Verification items for the finished model (mm, model axes). Face numbers are marked on the shaded views. A direction names the side the tool comes from. Round coordinates to 2 decimals unless told otherwise and drop trailing zeros. Write each loop counter-clockwise with the first axis right and the second up, starting at its lowest first coordinate (ties: lowest second). Pieces come first, ordered by that corner, then holes. Notation, with made-up numbers: (40, 73.5) -> (56, 73.5) arc R27 cw to (56, 111.5) -> close; hole circle Ø7 at (58, -4). An arc over 180 degrees is marked (long way). Answer as a JSON object with one key per item and string values. Group by question number.
(1) Set-up check for the marked faces 1, 2, 3, 4 and 5: record each of +Z, -Z, +X, -X, +Y, -Y from which the full face is reachable in a straight line by a thin tool's end or side.
(2) Sectioned sample at C-C on z = -1.5. Record the cut outline in (x, y).
(3) Gauge pin test, flat ends, axial feed: pin 1 Ø4.5 at (x, y) = (7.5, -19.5) entering from +Z; pin 2 Ø5 at (x, z) = (3, -15) entering from -Y; pin 3 Ø3 at (x, z) = (15.5, -7) entering from -Y; pin 4 Ø10 at (x, y) = (16.5, 34) entering from -Z. Record the tip position at first contact, or that the pin passes through.
(4) Scan lines: L1, parallel to X at y = 11, z = -17; L2, parallel to Y at x = 13, z = 2; L3, parallel to Z at x = 5.25, y = 18. Record each from-to range of solid material in increasing order. Write a range as from..to.
(5) Draft check along Z on the marked faces 6 and 7. Enter one of: released by +Z, released by -Z, zero draft, split by the parting line, or undercut.
(6) Sectioned sample at B-B on y = 49.5. Record the cut outline in (x, z), and give its area (3 significant figures).
(7) Sectioned sample at D-D on x = 16. Record the cut outline in (y, z), and give its area (3 significant figures).
```python
from build123d import *

# Parameters (mm, degrees)
BOSS_EXTRUDE1_DEPTH     = 50
CUT_EXTRUDE1_DEPTH      = 30
BOSS_EXTRUDE2_DEPTH     = 2
CUT_EXTRUDE2_DEPTH      = 2
CUT_EXTRUDE3_DEPTH      = 2
SKETCH9_W               = 3
SKETCH9_H               = 16.82
BOSS_EXTRUDE3_DEPTH     = 13
SKETCH10_W              = 4
SKETCH10_H              = 4
CUT_EXTRUDE4_DEPTH      = 15
BOSS_EXTRUDE4_DEPTH     = 8.82
FILLET1_R               = 1.5
SKETCH12_R              = 0.75
CUT_EXTRUDE5_DEPTH      = 57.090755147
CUT_EXTRUDE7_DEPTH      = 58.56944687
CUT_EXTRUDE7_DEPTH_BACK = 58.56944687
SKETCH15_R              = 0.75
BOSS_EXTRUDE5_DEPTH     = 7.6
CUT_EXTRUDE8_DEPTH      = 3
CUT_EXTRUDE9_DEPTH      = 3
SCALE1_SCALE            = 1.3


with BuildPart() as part:
    # Sketch1 → Boss-Extrude1 (new body)
    with BuildSketch(Plane(origin=(0, 0, 0), x_dir=(1, 0, 0), z_dir=(0, 1, 0))):
        Polygon((0, 0), (0, 16.82), (7.855052448, 23.008549995), (9.003996979, 21.550208451), (3, 16.82), (3, 0), (8.997095559, -4.738955219), (7.846023294, -6.199993425), align=None)
    extrude(amount=BOSS_EXTRUDE1_DEPTH)

    # Sketch2 → Cut-Extrude1 (cut, along a direction that is not the sketch's normal)
    with BuildSketch(Plane(origin=(0, 0, 0), x_dir=(0.7846023293722103, 0, 0.6199993425348946), z_dir=(-0.6199993425348946, 0, 0.7846023293722103))):
        Polygon((11.46, 50), (0, 37), (0, 50), align=None)
    extrude(amount=-CUT_EXTRUDE1_DEPTH, dir=(0, 0, 1), mode=Mode.SUBTRACT)

    # Sketch5 → Boss-Extrude2 (add, along a direction that is not the sketch's normal)
    with BuildSketch(Plane(origin=(-17.310263861, 11.972767428, 0), x_dir=(0, 0, 1), z_dir=(-0.8224425153975565, 0.568848230081223, 0))):
        Polygon((0, 30.43037307), (6.199993425, 44.223196672), (4.746003384, 46.236948917), (-21.566016526, 46.236948917), (-23.008549995, 44.239069366), (-16.82, 30.43037307), align=None)
    extrude(amount=BOSS_EXTRUDE2_DEPTH, dir=(0, 1, 0))

    # Sketch6 → Cut-Extrude2 (cut)
    with BuildSketch(Plane(origin=(0, 0, 0), x_dir=(0.7846023293722103, 0, 0.6199993425348946), z_dir=(-0.6199993425348946, 0, 0.7846023293722103))):
        Polygon((10, 50.343804538), (7, 0), (10, 0), align=None)
    extrude(amount=-CUT_EXTRUDE2_DEPTH, mode=Mode.SUBTRACT)

    # Sketch7 → Cut-Extrude3 (cut)
    with BuildSketch(Plane(origin=(-8.176434921, 0, -10.378250996), x_dir=(-0.7855052448151816, 0, 0.6188549994690533), z_dir=(-0.6188549994690533, 0, -0.7855052448151816))):
        Polygon((-20.409141091, 50.356858917), (-20.409141091, 0), (-17.409141091, 0), align=None)
    extrude(amount=-CUT_EXTRUDE3_DEPTH, mode=Mode.SUBTRACT)

    # Sketch9 → Boss-Extrude3 (add, along a direction that is not the sketch's normal)
    with BuildSketch(Plane.XZ):
        with Locations((1.5, -8.41)):
            Rectangle(SKETCH9_W, SKETCH9_H)
    extrude(amount=BOSS_EXTRUDE3_DEPTH, dir=(0.5000000000000012, -0.866025403784438, 0))

    # Sketch10 → Cut-Extrude4 (cut, along a direction that is not the sketch's normal)
    with BuildSketch(Plane(origin=(0, 0, 0), x_dir=(0, 0, 1), z_dir=(-0.8660254037844379, -0.5000000000000014, 0))):
        with Locations((-14.82, -11)):
            Rectangle(SKETCH10_W, SKETCH10_H)
        with Locations((-2, -11)):
            Rectangle(SKETCH10_W, SKETCH10_H)
    extrude(amount=-CUT_EXTRUDE4_DEPTH, dir=(-1, 0, 0), mode=Mode.SUBTRACT)

    # Sketch11 → Boss-Extrude4 (add)
    with BuildSketch(Plane(origin=(0, 0, -12.82), x_dir=(-1, 0, 0), z_dir=(0, 0, -1))):
        Polygon((-9.5, -11.258330249), (-7.25, -12.557368355), (-6.5, -11.258330249), align=None)
    extrude(amount=-BOSS_EXTRUDE4_DEPTH)

    # Fillet1
    # the kernel refuses this fillet: 1.5 mm, written as the material it takes off along each edge
    with BuildSketch(Plane(origin=(9.5, -11.258330249, -0.25), x_dir=(-0.8660254037844393, -0.49999999999999895, 0), z_dir=(0, 0, -1)), Plane(origin=(7.25, -12.557368355, -16.57), x_dir=(0.8660254037844389, 0.4999999999999996, 0), z_dir=(0, 0, 1))) as fillet1_piece_1:
        with BuildLine():
            CenterArc((FILLET1_R, FILLET1_R), FILLET1_R, 180, 90)
            Line((0, FILLET1_R), (0, 0))
            Line((0, 0), (FILLET1_R, 0))
        make_face()
    extrude(amount=16.32, mode=Mode.SUBTRACT)

    # Sketch12 → Cut-Extrude5 (cut, through all)
    with BuildSketch(Plane.XY.offset(-4)):
        with Locations((7.625, -10.608811196)):
            Circle(SKETCH12_R)
    extrude(amount=-CUT_EXTRUDE5_DEPTH, mode=Mode.SUBTRACT)

    # Sketch15 → Cut-Extrude7 (cut, two sides: drawn at the far end of the back side and taken through both)
    with BuildSketch(Plane.XY.offset(-CUT_EXTRUDE7_DEPTH_BACK)):
        with Locations(Location((5, 2, 0), (0, 0, 35.261867611))):
            Circle(SKETCH15_R)
    extrude(amount=CUT_EXTRUDE7_DEPTH + CUT_EXTRUDE7_DEPTH_BACK, mode=Mode.SUBTRACT)

    # Sketch17 → Boss-Extrude5 (add)
    with BuildSketch(Plane(origin=(8.991542695, 0, 0), x_dir=(0, 0, -1), z_dir=(1, 0, 0))):
        Polygon((-4.746003384, 52), (-4.717307032, 50), (21.531663082, 50), (21.566016526, 52), align=None)
    extrude(amount=BOSS_EXTRUDE5_DEPTH)

    # Sketch18 → Cut-Extrude8 (cut)
    with BuildSketch(Plane(origin=(0, 52, 0), x_dir=(1, 0, 0), z_dir=(0, 1, 0))):
        Polygon((8.991542695, 21.566016526), (16.591542695, 8.410006571), (16.591542695, 21.566016526), align=None)
    extrude(amount=-CUT_EXTRUDE8_DEPTH, mode=Mode.SUBTRACT)

    # Sketch19 → Cut-Extrude9 (cut)
    with BuildSketch(Plane(origin=(0, 52, 0), x_dir=(1, 0, 0), z_dir=(0, 1, 0))):
        Polygon((16.591542695, 8.410006571), (8.991542695, -4.746003384), (16.591542695, -4.746003384), align=None)
    extrude(amount=-CUT_EXTRUDE9_DEPTH, mode=Mode.SUBTRACT)


with BuildPart() as part_1:
    # Scale1: scaled about (3.445853057, 21.968382551, -8.406041901)
    add(part.part.scale(SCALE1_SCALE).moved(Location((-1.033755917, -6.590514765, 2.52181257))))


solid = part_1.part
```
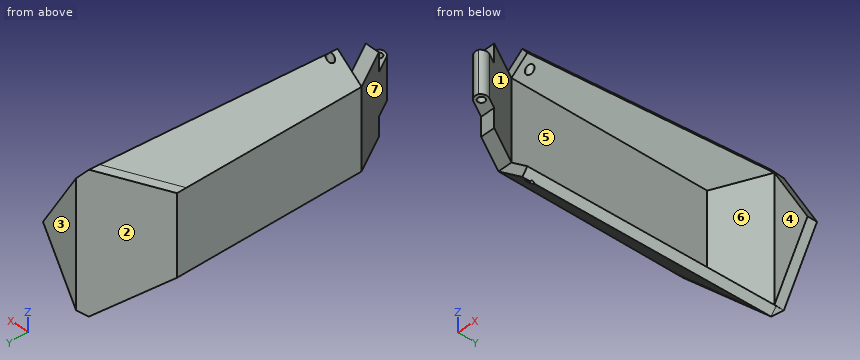
Computed values:
{
 "1": {"face 1": "+Z, -Z, +X", "face 2": "+Z, -Z, -X, +Y", "face 3": "+Z, -Z, +X, -X, +Y", "face 4": "+Z, -Z, +X, -Y", "face 5": "+X"},
 "2": {"outline": "(-1.03, -6.59) -> (4.82, -16.72) -> (8.72, -16.72) -> (2.87, -6.59) -> (2.87, 47.15) -> (10.66, 58.41) -> (16.54, 58.41) -> (16.54, 61.01) -> (10.66, 61.01) -> (-1.03, 44.11) -> close"},
 "3": {"pin 1": "z = -2.68", "pin 2": "y = -17.65", "pin 3": "y = 58.41", "pin 4": "through"},
 "4": {"L1": "-1.03..2.87", "L2": "58.41..61.01", "L3": "-24.29..-21.22, 4.41..7.49"},
 "5": {"face 6": "undercut", "face 7": "zero draft"},
 "6": {"outline": "(2.69, -22.28) -> (8.74, -27.04) -> (10.23, -25.15) -> (4.49, -20.63) -> (4.49, 3.81) -> (10.23, 8.34) -> (8.73, 10.24) -> (2.69, 5.47) -> close", "area": "83.2 mm2"},
 "7": {"outline": "(58.41, -16.26) -> (61.01, -16.26) -> (61.01, -0.56) -> (58.41, -0.56) -> close", "area": "40.8 mm2"}
}
